```python
from build123d import *

# Parameters (mm, degrees)
SKETCH1_R                                           = 33
BOSS_EXTRUDE1_DEPTH                                 = 8
SKETCH2_R                                           = 15.5
BOSS_EXTRUDE2_DEPTH                                 = 3
SKETCH4_R                                           = 3.05
CUT_EXTRUDE2_DEPTH                                  = 5
CHAMFER1_SIZE                                       = 0.5
CBORE_FOR_M6_HEX_SOCKET_THIN_HEAD_CA_2_COUNT        = 2
CBORE_FOR_M6_HEX_SOCKET_THIN_HEAD_CA_2_PITCH        = 50
CBORE_FOR_M6_HEX_SOCKET_THIN_HEAD_CA_3_A_COUNT      = 2
CBORE_FOR_M6_HEX_SOCKET_THIN_HEAD_CA_3_A_PITCH      = 50
CSK_FOR_M4_COUNTERSUNK_FLAT_HEAD_SCREW1_D           = 4.5
CSK_FOR_M4_COUNTERSUNK_FLAT_HEAD_SCREW1_CSINK_D     = 9.4
CSK_FOR_M4_COUNTERSUNK_FLAT_HEAD_SCREW1_CSINK_ANGLE = 90


with BuildPart() as part:
    # Sketch1 → Boss-Extrude1 (new body)
    with BuildSketch(Plane(origin=(0, 0, 0), x_dir=(1, 0, 0), z_dir=(0, 1, 0))):
        with Locations(Location((0, 0, 0), (0, 0, 270))):
            Circle(SKETCH1_R)
    extrude(amount=BOSS_EXTRUDE1_DEPTH)

    # Sketch2 → Boss-Extrude2 (add)
    with BuildSketch(Plane(origin=(0, 0, 0), x_dir=(-1, 0, 0), z_dir=(0, -1, 0))):
        with Locations(Location((0, 0, 0), (0, 0, 90))):
            Circle(SKETCH2_R)
    extrude(amount=BOSS_EXTRUDE2_DEPTH)

    # Sketch4 → Cut-Extrude2 (cut)
    with BuildSketch(Plane.XZ):
        with Locations(Location((-17.67766953, -17.67766953, 0), (0, 0, 270))):
            Circle(SKETCH4_R)
    extrude(amount=-CUT_EXTRUDE2_DEPTH, mode=Mode.SUBTRACT)

    # Chamfer1
    chamfer1_edges = [part.edges().sort_by_distance(p)[0] for p in [
        (0, -3, 15.5),
    ]]
    chamfer(chamfer1_edges, length=CHAMFER1_SIZE)

    # Sketch8 → CBORE for M6 Hex Socket Thin Head Cap Sc (revolve, cut)
    with BuildSketch(Plane(origin=(-25, 0, 0), x_dir=(0, 0, -1), z_dir=(1, 0, 0))):
        Polygon((0, 0), (0, 8), (3.3, 8), (3.3, 4.6), (5.5, 4.6), (5.5, 1), (6.5, 0), align=None)
    cbore_for_m6_hex_socket_thin_head_cap_sc = revolve(axis=Axis((-25, -6.35, 0), (0, 1, 0)), mode=Mode.SUBTRACT)

    # CBORE for M6 Hex Socket Thin Head Ca 2: CBORE for M6 Hex Socket Thin Head Cap Sc ×2
    with Locations(*[(i * CBORE_FOR_M6_HEX_SOCKET_THIN_HEAD_CA_2_PITCH, 0, 0) for i in range(1, CBORE_FOR_M6_HEX_SOCKET_THIN_HEAD_CA_2_COUNT)]):
        add(cbore_for_m6_hex_socket_thin_head_cap_sc, mode=Mode.SUBTRACT)

    # Sketch10 → CBORE for M6 Hex Socket Thin Head Ca 3 (revolve, cut)
    with BuildSketch(Plane(origin=(0, 8, -25), x_dir=(0, 0, 1), z_dir=(1, 0, 0))):
        Polygon((0, 0), (0, 11), (3.3, 11), (3.3, 4.6), (5.5, 4.6), (5.5, 1), (6.5, 0), align=None)
    cbore_for_m6_hex_socket_thin_head_ca_3 = revolve(axis=Axis((0, 14.35, -25), (0, -1, 0)), mode=Mode.SUBTRACT)

    # CBORE for M6 Hex Socket Thin Head Ca 3 a: CBORE for M6 Hex Socket Thin Head Ca 3 ×2
    with Locations(*[(0, 0, i * CBORE_FOR_M6_HEX_SOCKET_THIN_HEAD_CA_3_A_PITCH) for i in range(1, CBORE_FOR_M6_HEX_SOCKET_THIN_HEAD_CA_3_A_COUNT)]):
        add(cbore_for_m6_hex_socket_thin_head_ca_3, mode=Mode.SUBTRACT)

    # CSK for M4 Countersunk Flat Head Screw1 (through all)
    with Locations(Plane(origin=(0, -3, 0), x_dir=(-1, 0, 0), z_dir=(0, -1, 0))):
        with Locations((0, 0)):
            CounterSinkHole(CSK_FOR_M4_COUNTERSUNK_FLAT_HEAD_SCREW1_D / 2, CSK_FOR_M4_COUNTERSUNK_FLAT_HEAD_SCREW1_CSINK_D / 2, counter_sink_angle=CSK_FOR_M4_COUNTERSUNK_FLAT_HEAD_SCREW1_CSINK_ANGLE)


solid = part.part
```
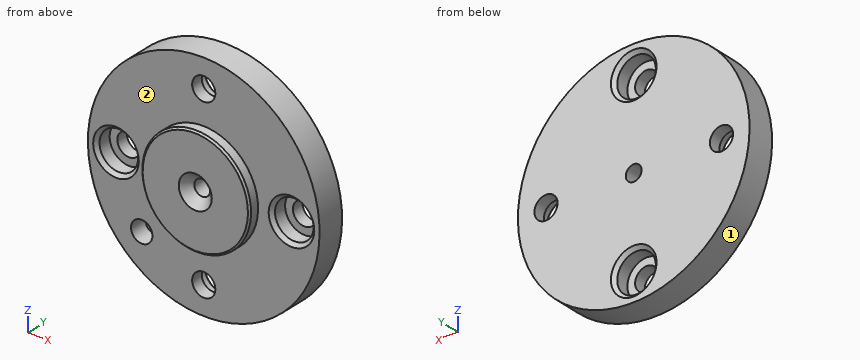
Source: CAD feature listing. Evaluate the final solid. Frame: model axes, mm. Face numbers are marked on the shaded views. A direction names the side the tool comes from. Coordinates: 2 decimals unless noted, no trailing zeros. Write each loop counter-clockwise with the first axis right and the second up, starting at its lowest first coordinate (ties: lowest second). Pieces come first, ordered by that corner, then holes. Notation, with made-up numbers: (68.5, 45.25) -> (73.5, 45.25) arc R9 ccw to (73.5, 62.25) -> close; hole circle Ø3 at (43, 4.5). An arc over 180 degrees is marked (long way). Return JSON: item names as keys, results as strings. Group by question number.
1) Section query B-B, the plane z = 25. Return loops of the section in (x, y), plus the area to 3 significant figures.
2) Contact query for flat-ended pins moving along their axis: P1, Ø17.5, axis at x = 25, z = 0, coming from the -Y side; P2, Ø3, axis at x = -18, z = -18.5, coming from the -Y side; P3, Ø10.5, axis at x = 25, z = 0, coming from the -Y side; P4, Ø12, axis at x = 1.5, z = -26, coming from the +Y side. Output: stop coordinate, or through.
3) Section query A-A, the plane x = 25. Return loops of the section in (y, z).
4) Section query C-C, the plane x = 0. State how many separate pieces and enclosed holes the cut face has, plus the area to 3 significant figures.
5) Ray query, line 1 along X through (y, z) = (7, 2); line 2 along X through (y, z) = (-0.25, -1.5); line 3 along Y through (x, z) = (16.5, -9.5). Return the intervals inside material, ascending.
6) Set-up query: the marked faces 1 and 2. Return all of +Z, -Z, +X, -X, +Y, -Y with unobstructed straight access to the full face (end or side cutting, diameter ignored); none if empty.
From the geometry:
{
 "1": {"outline": "(-21.54, 0) -> (-3.3, 0) -> (-3.3, 3.4) -> (-5.5, 3.4) -> (-5.5, 7) -> (-6.5, 8) -> (-21.54, 8) -> close; (3.3, 0) -> (21.54, 0) -> (21.54, 8) -> (6.5, 8) -> (5.5, 7) -> (5.5, 3.4) -> (3.3, 3.4) -> close", "area": "271 mm²"},
 "2": {"P1": "y = 0", "P2": "y = 5", "P3": "y = 4.6", "P4": "y = 8"},
 "3": {"outline": "(0, -21.54) -> (8, -21.54) -> (8, -3.3) -> (4.6, -3.3) -> (4.6, -5.5) -> (1, -5.5) -> (0, -6.5) -> close; (0, 6.5) -> (1, 5.5) -> (4.6, 5.5) -> (4.6, 3.3) -> (8, 3.3) -> (8, 21.54) -> (0, 21.54) -> close"},
 "4": {"separate pieces": "4", "enclosed holes": "0", "area": "417 mm²"},
 "5": {"line 1": "-32.94 to -27.62, -22.38 to -1.03, 1.03 to 22.38, 27.62 to 32.94", "line 2": "-15.43 to -1.68, 1.68 to 15.43", "line 3": "0 to 8"},
 "6": {"face 1": "+Y, -Y", "face 2": "-Y"}
}
